Build history of the part. All positions in model axes, mm. Round coordinates to 2 decimals unless told otherwise and drop trailing zeros. Write each loop counter-clockwise with the first axis right and the second up, starting at its lowest first coordinate (ties: lowest second). Pieces come first, ordered by that corner, then holes. Notation, with made-up numbers: (39, -11) - (80, -11) arc R17 ccw to (80, 4) - close; hole circle Ø7 at (62, 14). An arc over 180 degrees is marked (long way). Answer as a JSON object with one key per item and string values. Group by question number.
Item 1: Slice it at C-C, the plane z = 59. Give the number of separate pieces and of enclosed holes in the cut face, then the cut area to 3 significant figures.
Item 2: Slice it at D-D, the plane x = 31. List the corners of the cut face in (y, z).
Item 3: Slice it at B-B, the plane y = -33.5. List the corners of the cut face in (x, z), then the cut area to 3 significant figures.
Item 4: Flat gauge pins, fed straight in: pin 1 (1 mm diameter, centred on y = -32, z = 32.5, fed in from -X); pin 2 (4 mm diameter, centred on x = -67.5, y = 22.5, fed in from +Z). Where does each tip first touch, or does it go through?
Item 5: Probe line 1 (X direction, y = -1, z = 44); line 2 (Z direction, x = 10, y = -31.5); line 3 (X direction, y = -36, z = 36.5). List the from-to ranges inside material, lowest first. Write a range as from..to.
Item 6: Slice it at A-A, the plane z = 29. List the corners of the cut face in (x, y), then the cut area to 3 significant figures.
from build123d import *

# Parameters (mm, degrees)
BOSS_EXTRUDE1_DEPTH  = 57.15
CUT_EXTRUDE1_START   = -16.000000004
SKETCH3_R            = 3.499999985
CUT_EXTRUDE1_DEPTH   = 105.568182472
CUT_SWEEP1_PROFILE_R = 1.3462
CUT_SWEEP2_START     = 54.2798
CUT_SWEEP2_OUTLINE_R = 3.175
CUT_SWEEP2_DEPTH     = 11.070212874


# Read off the part's stored shape, not the designer's step: Cut-Sweep2
with BuildPart() as part:
    # Sketch1 → Boss-Extrude1 (new, symmetric)
    with BuildSketch(Plane(origin=(0, 0, 0), x_dir=(1, 0, 0), z_dir=(0, 1, 0))):
        with BuildLine():
            Line((-44.258055055, -25.5524), (-84.849935901, -48.988133333))
            Line((-84.849935901, -48.988133333), (-59.186716436, -63.8048))
            Line((-59.186716436, -63.8048), (0, -63.8048))
            Line((0, -63.8048), (0, -51.1048))
            ThreePointArc((0, -51.1048), (-25.5524, -44.258055055), (-44.258055055, -25.5524))
        make_face()
        with BuildLine():
            Line((0, -51.1048), (0, -63.8048))
            Line((0, -63.8048), (59.186716436, -63.8048))
            Line((59.186716436, -63.8048), (84.849935901, -48.988133333))
            Line((84.849935901, -48.988133333), (44.258055055, -25.5524))
            ThreePointArc((44.258055055, -25.5524), (25.5524, -44.258055055), (0, -51.1048))
        make_face()
    extrude(amount=BOSS_EXTRUDE1_DEPTH, both=True)

    # Sketch2 → Cut-Revolve7 (revolve, cut)
    with BuildSketch(Plane(origin=(0, 0, 0), x_dir=(1, 0, 0), z_dir=(0, 1, 0)), mode=Mode.PRIVATE) as cut_revolve7_sk:
        Polygon((-43.878504985, -64.929800036), (-44.528024059, -63.8048), (-48.569475926, -63.8048), (-47.770256416, -65.189088798), (-46.909593885, -66.679800029), align=None)
        Polygon((-48.569475926, -63.8048), (-44.528024059, -63.8048), (-51.024306947, -52.552907978), (-54.055395847, -54.30290797), align=None)
        Polygon((-54.055395847, -54.30290797), (-51.024306947, -52.552907978), (-61.024306886, -35.232400008), (-64.055395786, -36.9824), align=None)
    cut_revolve7 = revolve(cut_revolve7_sk.sketch.rotate(Axis((-64.055395786, 0, 36.9824), (0.4999999999999998, 0, 0.8660254037844388)), 180), axis=Axis((-64.055395786, 0, 36.9824), (0.4999999999999998, 0, 0.8660254037844388)), mode=Mode.SUBTRACT)

    # Sketch2<7> → Cut-Revolve8 (revolve, cut)
    with BuildSketch(Plane(origin=(0, 0, 0), x_dir=(1, 0, 0), z_dir=(0, 1, 0)), mode=Mode.PRIVATE) as cut_revolve8_sk:
        Polygon((-44.528024059, -63.8048), (-41.929947764, -63.8048), (-49.075749726, -51.427907942), (-51.024306947, -52.552907978), align=None)
    revolve(cut_revolve8_sk.sketch.rotate(Axis((-64.055395786, 0, 36.9824), (0.4999999999999998, 0, 0.8660254037844388)), 180), axis=Axis((-64.055395786, 0, 36.9824), (0.4999999999999998, 0, 0.8660254037844388)), mode=Mode.SUBTRACT)

    # Mirror1: Cut-Revolve7 across plane
    add(cut_revolve7.mirror(Plane(origin=(0, 0, 0), x_dir=(0, 0, 1), z_dir=(1, 0, 0))), mode=Mode.SUBTRACT)

    # Sketch3 → Cut-Extrude1 (cut, through all)
    with BuildSketch(Plane(origin=(0, 0, 0), x_dir=(-0.8660254037844386, 0, -0.5000000000000001), z_dir=(0.5000000000000001, 0, -0.8660254037844386)).offset(CUT_EXTRUDE1_START)):
        Polygon((-76.995888937, 5.250000041), (-80.026977874, 0), (-76.995888937, -5.250000041), (-70.933711063, -5.250000041), (-67.902622126, 0), (-70.933711063, 5.250000041), align=None)
        with Locations(Location((-73.9648, 0, 0), (0, 0, 180))):
            Circle(SKETCH3_R, mode=Mode.SUBTRACT)
    extrude(amount=-CUT_EXTRUDE1_DEPTH, mode=Mode.SUBTRACT)

    # Cut-Sweep1: sweep along a path in Sketch4
    with BuildLine(Plane(origin=(0, 0, 0), x_dir=(1, 0, 0), z_dir=(0, 1, 0))) as cut_sweep1_path:
        Line((0, 0), (9.429525456, -53.454473505))
    # Cut-Sweep1 profile (on start of the path) → Cut-Sweep1 (sweep, cut)
    with BuildSketch(Plane(origin=(0, 0, 0), x_dir=(0.984794960650155, 0, -0.17372071113733015), z_dir=(0.17372071113733015, 0, 0.984794960650155))):
        Circle(CUT_SWEEP1_PROFILE_R)
    sweep(path=cut_sweep1_path.line, mode=Mode.SUBTRACT)

    # Cut-Sweep2 outline → Cut-Sweep2 (cut)
    with BuildSketch(Plane(origin=(0, 0, 0), x_dir=(0.984794960650155, 0, -0.17372071113733004), z_dir=(0.17372071113733, 0, 0.984794960650155)).offset(CUT_SWEEP2_START)):
        Circle(CUT_SWEEP2_OUTLINE_R)
    extrude(amount=CUT_SWEEP2_DEPTH, mode=Mode.SUBTRACT)


solid = part.part
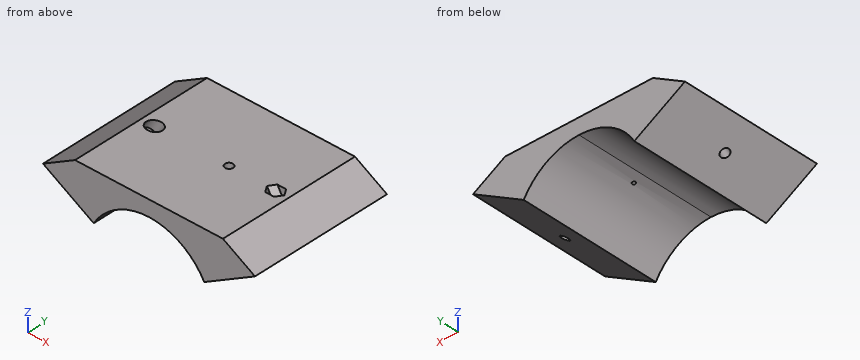
Geometry says:
{
 "1": {"separate pieces": "1", "enclosed holes": "3", "area": "15,200 mm^2"},
 "2": {"outline": "(-57.15, 40.63) - (57.15, 40.63) - (57.15, 63.8) - (-57.15, 63.8) - close"},
 "3": {"outline": "(-84.85, 48.99) - (-44.26, 25.55) arc R51.1 cw to (44.26, 25.55) - (84.85, 48.99) - (59.19, 63.8) - (-59.19, 63.8) - close", "area": "3,560 mm^2"},
 "4": {"pin 1": "stops at x = -57.16", "pin 2": "stops at z = 60.16"},
 "5": {"line 1": "x = -76.21..-63.88, -56.13..-25.99, 25.99..56.13, 63.88..76.21", "line 2": "z = 50.12..63.8", "line 3": "x = -63.22..-35.77, 35.77..63.22"},
 "6": {"outline": "(-50.23, -57.15) - (-42.08, -57.15) - (-42.08, 57.15) - (-50.23, 57.15) - close; (42.08, -57.15) - (50.23, -57.15) - (50.23, 57.15) - (42.08, 57.15) - close", "area": "1,860 mm^2"}
}
